Could you check a few things on this model? Use its own coordinates, in mm. Face numbers are marked on the shaded views. A direction names the side the tool comes from. Round coordinates to 2 decimals unless told otherwise and drop trailing zeros. Loops run counter-clockwise (first coordinate to the right, second up) from the corner with the lowest first, then second, coordinate; pieces in that order, holes last.
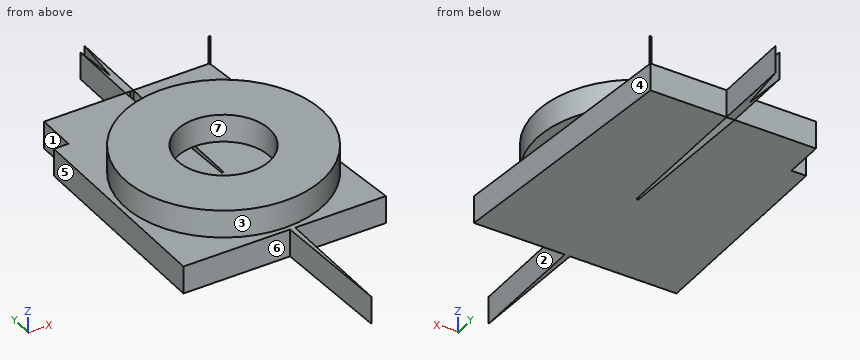
from build123d import *

# Parameters (mm, degrees)
F1_DEPTH = 25.4
F2_R     = 0.6873607635
F2_R_2   = 90.9704794281
F2_R_3   = 42.2453138018
F3_DEPTH = 25.4


with BuildPart() as f1:
    # F0 (on Top) → F1 (new body)
    with BuildSketch(Plane.XY):
        Polygon((0, 89.7069421623), (0, 0), (-1.810804775, 0), (2.1516823224, -95.0307697058), (6.8773888052, -95.0307697058), (6.8773888052, -13.3527815342), align=None)
        Polygon((2.1516823224, -95.0307697058), (-1.810804775, 0), (-95.6487208605, 0), (-95.6487208605, -95.0307697058), align=None)
        Polygon((-95.6487208605, 0), (-1.810804775, 0), (-5.859600791, 97.1006825566), (-82.1735113859, 97.1006825566), (-95.6487208605, 97.1006825566), align=None)
        Polygon((0, 97.1006825566), (0, 89.7069421623), (6.8773888052, -13.3527815342), (6.8773888052, -95.0307697058), (90.1318565011, -95.0307697058), (70.0762048364, 133.9463293552), (0, 133.6299567875), (0, 133.2589685917), align=None)
        Polygon((-82.1735113859, 97.1006825566), (-5.859600791, 97.1006825566), (-7.3672886938, 133.2589685917), (-82.1735113859, 133.2589685917), align=None)
        Polygon((6.8773888052, -95.0307697058), (2.1516823224, -95.0307697058), (6.8773888052, -208.3655297756), align=None)
        Polygon((-7.3672886938, 133.5966957391), (-7.3672886938, 133.2589685917), (-7.3332104262, 133.596849592), align=None)
        Polygon((-82.1735113859, 133.2589685917), (-7.3672886938, 133.2589685917), (-7.3672886938, 133.5966957391), align=None)
        Polygon((-2.9063169225, 133.2589685917), (0, 133.2589685917), (0, 133.6299567875), (-2.9301909404, 133.6167278743), align=None)
        Polygon((-7.3672886938, 133.5966957391), (-7.3332104262, 133.596849592), (-4.6826064537, 159.8771973232), (-7.3672886938, 200.1079618931), align=None)
        Polygon((-4.6826064537, 159.8771973232), (-7.3332104262, 133.596849592), (-2.9301909404, 133.6167278743), align=None)
        Polygon((-2.9301909404, 133.6167278743), (0, 133.6299567875), (0, 206.3045501709), (-4.6826064537, 159.8771973232), align=None)
    extrude(amount=F1_DEPTH)

    # F2 (on face) → F3 (join)
    with BuildSketch(Plane.XY.offset(25.4)):
        with Locations((70.0762048364, 133.9463293552)):
            Circle(F2_R)
        Circle(F2_R_2)
        Circle(F2_R_3, mode=Mode.SUBTRACT)
    extrude(amount=F3_DEPTH)


solid = f1.part
Item 1: If I drill on line 1 along X through (y, z) = (0, 33.75); line 2 along X through (y, z) = (46, 24.5), over which ranges is the centre line in solid material (lowest first)?
Results list:
line 1: x = -90.97 to -42.25, 42.25 to 90.97
line 2: x = -95.65 to -3.73, 0 to 77.78
Item 2: If we section it at C-C, the plane z = 20.5: Please give me the cut outline in (x, y).
Results list:
outline: (-95.65, -95.03) - (2.15, -95.03) - (6.88, -208.37) - (6.88, -95.03) - (90.13, -95.03) - (70.08, 133.95) - (0, 133.63) - (0, 206.3) - (-4.68, 159.88) - (-7.37, 200.11) - (-7.37, 133.6) - (-82.17, 133.26) - (-82.17, 97.1) - (-95.65, 97.1) - close; hole (-7.37, 133.26) - (-1.81, 0) - (0, 0) - (0, 133.26) - (-2.91, 133.26) - (-2.93, 133.62) - (-7.33, 133.6) - close
Item 3: If we section it at B-B, the plane y = 178: Please give me the cut outline in (x, z), then the cut area to 3 significant figures.
Results list:
outline: (-7.37, 0) - (-5.89, 0) - (-5.89, 25.4) - (-7.37, 25.4) - close; (-2.85, 0) - (0, 0) - (0, 25.4) - (-2.85, 25.4) - close
area: 110 mm2
Item 4: For the marked faces 1, 2, 3 and 4, which set-ups out of +Z, -Z, +X, -X, +Y, -Y let a thin tool reach every point of the face, with its end or its side?
Results list:
face 1: +Z, -Z, -X, +Y
face 2: +Z, -Z, +X, -Y
face 3: +Z
face 4: -Z, +X, +Y
Item 5: Will these pins go through, and if not, where does the flat tip stop? pin 1 (8 mm diameter, centred on x = 55.5, z = 15, fed in from +Y); pin 2 (20.5 mm diameter, centred on x = -55.5, z = 13.5, fed in from -Y); pin 3 (15 mm diameter, centred on x = -88.5, z = 12.5, fed in from +Y); pin 4 (8 mm diameter, centred on y = 146, z = 32, fed in from -X).
Results list:
pin 1: stops at y = 133.9
pin 2: stops at y = -95.03
pin 3: stops at y = 133.26
pin 4: passes through
Item 6: We'd pull the mould along Y, two halves only. Please class the marked faces 5, 6 and 7: released by +Y, released by -Y, zero draft, split by the parting line, or undercut.
Results list:
face 5: zero draft
face 6: released by -Y
face 7: undercut
Item 7: If we section it at A-A, the plane z = 42: Please give me the cut outline in (x, y).
Results list:
outline: circle Ø181.94 at (0, 0); circle Ø1.37 at (70.08, 133.95); hole circle Ø84.49 at (0, 0)
Item 8: If we section it at D-D, the plane x = -53: Please give me the cut outline in (y, z).
Results list:
outline: (-95.03, 0) - (133.39, 0) - (133.39, 25.4) - (73.94, 25.4) - (73.94, 50.8) - (-73.94, 50.8) - (-73.94, 25.4) - (-95.03, 25.4) - close
